CAD build for the part. Positions are in the model's coordinates, mm. A direction names the side the tool comes from. Give positions to 0.01 mm unless a question says otherwise; leave off trailing zeros. Loops run counter-clockwise (first coordinate to the right, second up) from the corner with the lowest first, then second, coordinate; pieces in that order, holes last.
```python
from build123d import *

# Parameters (mm, degrees)
SKETCH1_W               = 168.379590863
SKETCH1_H               = 126.39
BOSS_EXTRUDE1_DEPTH     = 70
SKETCH2_W               = 168.379590863
SKETCH2_H               = 126.39
BOSS_EXTRUDE2_DEPTH     = 4
SKETCH3_W               = 142.779590863
SKETCH3_H               = 96.34
CUT_EXTRUDE1_DEPTH      = 4
FILLET1_R               = 5
FILLET4_R               = 2
FILLET5_R               = 2
SKETCH4_W               = 10
SKETCH4_H               = 10
CUT_EXTRUDE2_DEPTH      = 195
SKETCH6_R               = 2
CUT_EXTRUDE3_DEPTH      = 195
SKETCH8_R               = 2
CUT_EXTRUDE4_DEPTH      = 195
CUT_EXTRUDE5_DEPTH      = 134.542245944
CUT_EXTRUDE5_DEPTH_BACK = 134.542245944
SKETCH12_W              = 87.181234027
SKETCH12_H              = 80.365226026
SKETCH14_W              = 5
SKETCH14_H              = 2
BOSS_EXTRUDE4_DEPTH     = 15
SKETCH17_W              = 2
SKETCH17_H              = 2
BOSS_EXTRUDE5_DEPTH     = 15
SKETCH18_W              = 1.5
SKETCH18_H              = 5
BOSS_EXTRUDE8_DEPTH     = 15
SKETCH19_W              = 1.5
SKETCH19_H              = 5
BOSS_EXTRUDE9_DEPTH     = 15


with BuildPart() as part:
    # Sketch1 → Boss-Extrude1 (new body)
    with BuildSketch(Plane(origin=(0, 0, 0), x_dir=(1, 0, 0), z_dir=(0, 1, 0))):
        with Locations((4.455204569, -8.048213198)):
            Rectangle(SKETCH1_W, SKETCH1_H)
        Polygon((-76.734590863, 32.146786802), (-76.734590863, 52.146786802), (85.645, 52.146786802), (85.645, -68.243213198), (60.555409137, -68.243213198), (-76.734590863, -68.243213198), align=None, mode=Mode.SUBTRACT)
    extrude(amount=BOSS_EXTRUDE1_DEPTH)

    # Sketch2 → Boss-Extrude2 (add)
    with BuildSketch(Plane(origin=(0, 0, 0), x_dir=(-1, 0, 0), z_dir=(0, -1, 0))):
        with Locations((-4.455204569, -8.048213198)):
            Rectangle(SKETCH2_W, SKETCH2_H)
    extrude(amount=BOSS_EXTRUDE2_DEPTH)

    # Sketch3 → Cut-Extrude1 (cut)
    with BuildSketch(Plane(origin=(0, 0, 0), x_dir=(1, 0, 0), z_dir=(0, 1, 0))):
        with Locations((9.755204569, 0.476786802)):
            Rectangle(SKETCH3_W, SKETCH3_H)
    extrude(amount=-CUT_EXTRUDE1_DEPTH, mode=Mode.SUBTRACT)

    # Fillet1
    fillet1_edges = [part.edges().sort_by_distance(p)[0] for p in [
        (-79.734590863, 33, -55.146786802),
        (88.645, 33, -55.146786802),
        (88.645, 33, 71.243213198),
        (-79.734590863, 33, 71.243213198),
    ]]
    fillet(fillet1_edges, radius=FILLET1_R)

    # Fillet4
    fillet4_edges = [part.edges().sort_by_distance(p)[0] for p in [
        (4.455204569, -4, 71.243213198),
        (-79.734590863, -4, 8.048213198),
        (4.455204569, -4, -55.146786802),
        (88.645, -4, 8.048213198),
        (87.180533906, -4, 69.778747104),
        (87.180533906, -4, -53.682320708),
        (-78.270124769, -4, -53.682320708),
        (-78.270124769, -4, 69.778747104),
    ]]
    fillet(fillet4_edges, radius=FILLET4_R)

    # Fillet5
    fillet5_edges = [part.edges().sort_by_distance(p)[0] for p in [
        (81.145, -4, -0.476786802),
        (9.755204569, -4, 47.693213198),
        (-61.634590863, -4, -0.476786802),
        (9.755204569, -4, -48.646786802),
    ]]
    fillet(fillet5_edges, radius=FILLET5_R)

    # Sketch4 → Cut-Extrude2 (cut)
    with BuildSketch(Plane.ZY.offset(79.734590863)):
        with Locations((5.00870497, 36.749697215)):
            Rectangle(SKETCH4_W, SKETCH4_H)
    extrude(amount=-CUT_EXTRUDE2_DEPTH, mode=Mode.SUBTRACT)

    # Sketch6 → Cut-Extrude3 (cut)
    with BuildSketch(Plane(origin=(88.645, 0, 0), x_dir=(0, 0, -1), z_dir=(1, 0, 0))):
        with Locations((-7.57558331, 65)):
            Circle(SKETCH6_R)
    extrude(amount=-CUT_EXTRUDE3_DEPTH, mode=Mode.SUBTRACT)

    # Sketch8 → Cut-Extrude4 (cut)
    with BuildSketch(Plane(origin=(0, 0, -55.146786802), x_dir=(-1, 0, 0), z_dir=(0, 0, -1))):
        with Locations((-43.645, 65)):
            Circle(SKETCH8_R)
        with Locations((34.734590863, 65)):
            Circle(SKETCH8_R)
    extrude(amount=-CUT_EXTRUDE4_DEPTH, mode=Mode.SUBTRACT)

    # Sketch12 → Cut-Extrude5 (cut, two sides: drawn at the far end of the back side and taken through both)
    with BuildSketch(Plane.XY.offset(-CUT_EXTRUDE5_DEPTH_BACK)):
        with Locations((48.045821583, 29.817386987)):
            Rectangle(SKETCH12_W, SKETCH12_H)
    extrude(amount=CUT_EXTRUDE5_DEPTH + CUT_EXTRUDE5_DEPTH_BACK, mode=Mode.SUBTRACT)

    # Sketch14 → Boss-Extrude4 (add)
    with BuildSketch(Plane(origin=(4.455204569, 0, 0), x_dir=(0, 0, -1), z_dir=(1, 0, 0))):
        with Locations((-55.193213198, -1)):
            Rectangle(SKETCH14_W, SKETCH14_H)
        with Locations((-65.193213198, -1)):
            Rectangle(SKETCH14_W, SKETCH14_H)
    extrude(amount=BOSS_EXTRUDE4_DEPTH)

    # Sketch17 → Boss-Extrude5 (add)
    with BuildSketch(Plane(origin=(4.455204569, 0, 0), x_dir=(0, 0, -1), z_dir=(1, 0, 0))):
        with Locations((51.146786802, -1)):
            Rectangle(SKETCH17_W, SKETCH17_H)
    extrude(amount=BOSS_EXTRUDE5_DEPTH)

    # Sketch18 → Boss-Extrude8 (add)
    with BuildSketch(Plane(origin=(4.455204569, 0, 0), x_dir=(0, 0, -1), z_dir=(1, 0, 0))):
        with Locations((-68.993213198, 62.5)):
            Rectangle(SKETCH18_W, SKETCH18_H)
        with Locations((-68.993213198, 52.5)):
            Rectangle(SKETCH18_W, SKETCH18_H)
        with Locations((-68.993213198, 42.5)):
            Rectangle(SKETCH18_W, SKETCH18_H)
        with Locations((-68.993213198, 32.5)):
            Rectangle(SKETCH18_W, SKETCH18_H)
        with Locations((-68.993213198, 22.5)):
            Rectangle(SKETCH18_W, SKETCH18_H)
        with Locations((-68.993213198, 12.5)):
            Rectangle(SKETCH18_W, SKETCH18_H)
    extrude(amount=BOSS_EXTRUDE8_DEPTH)

    # Sketch19 → Boss-Extrude9 (add)
    with BuildSketch(Plane(origin=(4.455204569, 0, 0), x_dir=(0, 0, -1), z_dir=(1, 0, 0))):
        with Locations((52.896786802, 57.5)):
            Rectangle(SKETCH19_W, SKETCH19_H)
        with Locations((52.896786802, 67.5)):
            Rectangle(SKETCH19_W, SKETCH19_H)
        with Locations((52.896786802, 47.5)):
            Rectangle(SKETCH19_W, SKETCH19_H)
        with Locations((52.896786802, 37.5)):
            Rectangle(SKETCH19_W, SKETCH19_H)
        with Locations((52.896786802, 27.5)):
            Rectangle(SKETCH19_W, SKETCH19_H)
        with Locations((52.896786802, 17.5)):
            Rectangle(SKETCH19_W, SKETCH19_H)
    extrude(amount=BOSS_EXTRUDE9_DEPTH)


solid = part.part
```
1. Probe line 1 along Z through (x, y) = (-18.5, 65.5); line 2 along Y through (x, z) = (-74.5, -12); line 3 along Z through (x, y) = (10.5, 58). List the from-to ranges inside material, lowest first.
Responses:
line 1: z = -55.15 to -52.15, 68.24 to 71.24
line 2: y = -4 to 0
line 3: z = -53.65 to -52.15
2. Saw through at A-A, the plane x = -12. List the corners of the cut face in (y, z), and give its area (3 significant figures).
Responses:
outline: (-4, -53.15) arc R2 ccw to (-2, -55.15) - (70, -55.15) - (70, -52.15) - (0, -52.15) - (0, -48.65) - (-2, -48.65) arc R2 ccw to (-4, -50.65) - close; (-4, 49.69) arc R2 ccw to (-2, 47.69) - (0, 47.69) - (0, 68.24) - (70, 68.24) - (70, 71.24) - (-2, 71.24) arc R2 ccw to (-4, 69.24) - close
area: 537 mm2
3. Pull direction Z, two halves, no side cores. Call faces 1 (the face through (-78.23, 34.5, -53.72)), 2 (the face through (-35, 35, 71.243)), 3 (the face through (-35.81, 66.686, 69.722)), 4 (the face through (-78, 31.75, 5)): released by +Z, released by -Z, zero draft, split by the parting line, or undercut.
Responses:
face 1: released by -Z
face 2: released by +Z
face 3: zero draft
face 4: undercut
4. Tool access for faces 5 (the face through (12, 27, -53.647)), 6 (the face through (12, 32, 69.743)), 7 (the face through (-78, 37, 10.009)), 8 (the face through (-35, 35, -55.147)), 9 (the face through (-28, 35, 68.243)): list every direction of +Z, -Z, +X, -X, +Y, -Y with a clear straight run to the whole face (end or side of a thin tool).
Responses:
face 5: -Z, +X, +Y, -Y
face 6: +Z, +X, +Y, -Y
face 7: +X, -X
face 8: -Z, +X, -X, +Y, -Y
face 9: +X, +Y
5. Drop flat-ended pins along their axis: pin 1 (5 mm diameter, centred on x = -34.73, y = 65, fed in from -Z); pin 2 (5 mm diameter, centred on y = 11, z = 45, fed in from +X); pin 3 (1.6 mm diameter, centred on x = 9, z = 69, fed in from -Y); pin 4 (0.8 mm diameter, centred on x = 14, z = -53, fed in from -Y). Give the stop position or say it passes through.
Responses:
pin 1: stops at z = -55.15
pin 2: stops at x = -76.73
pin 3: stops at y = 10
pin 4: stops at y = 15
6. Saw through at D-D, the plane x = -73. List the corners of the cut face in (y, z), and give its area (3 significant figures).
Responses:
outline: (-4, -53.15) arc R2 ccw to (-2, -55.15) - (70, -55.15) - (70, -52.15) - (0, -52.15) - (0, 68.24) - (70, 68.24) - (70, 71.24) - (-2, 71.24) arc R2 ccw to (-4, 69.24) - close
area: 924 mm2
7. Saw through at B-B, the plane z = -28. List the corners of the cut face in (x, y).
Responses:
outline: (-79.73, -2) arc R2 ccw to (-77.73, -4) - (-63.63, -4) arc R2 ccw to (-61.63, -2) - (-61.63, 0) - (-76.73, 0) - (-76.73, 70) - (-79.73, 70) - close
8. Saw through at C-C, the plane y = 7. List the corners of the cut face in (x, z), and give its area (3 significant figures).
Responses:
outline: (-79.73, -50.15) arc R5 ccw to (-74.73, -55.15) - (4.46, -55.15) - (4.46, -52.15) - (-76.73, -52.15) - (-76.73, 68.24) - (4.46, 68.24) - (4.46, 71.24) - (-74.73, 71.24) arc R5 ccw to (-79.73, 66.24) - close
area: 856 mm2
